```python
from build123d import *

# Parameters (mm, degrees)
SKETCH1_R           = 10
BOSS_EXTRUDE1_DEPTH = 10
SKETCH2_R           = 100
BOSS_EXTRUDE2_DEPTH = 10
SKETCH3_R           = 7.5
BOSS_EXTRUDE3_DEPTH = 10


with BuildPart() as part:
    # Sketch1 → Boss-Extrude1 (new body)
    with BuildSketch(Plane(origin=(0, 0, 0), x_dir=(1, 0, 0), z_dir=(0, 1, 0))):
        with BuildLine():
            ThreePointArc((48.173076923, 57.483516418), (-75, 0), (48.173076923, -57.483516418))
            ThreePointArc((48.173076923, -57.483516418), (30, 0), (48.173076923, 57.483516418))
        make_face()
        with Locations(Location((0, 0, 0), (0, 0, 270))):
            Circle(SKETCH1_R, mode=Mode.SUBTRACT)
    extrude(amount=BOSS_EXTRUDE1_DEPTH)

    # Sketch2 → Boss-Extrude2 (add)
    with BuildSketch(Plane.XZ):
        with Locations(Location((0, 0, 0), (0, 0, 270))):
            Circle(SKETCH2_R)
    extrude(amount=BOSS_EXTRUDE2_DEPTH)

    # Sketch3 → Boss-Extrude3 (add)
    with BuildSketch(Plane(origin=(0, 0, 0), x_dir=(1, 0, 0), z_dir=(0, 1, 0))):
        with Locations(Location((80, 0, 0), (0, 0, 90))):
            Circle(SKETCH3_R)
    extrude(amount=BOSS_EXTRUDE3_DEPTH)


solid = part.part
```
Verification items for the finished model (mm, model axes). A direction names the side the tool comes from. Round coordinates to 2 decimals unless told otherwise and drop trailing zeros. Order: outer loops, then holes, each group sorted by start corner. A loop starts at its lowest first (then second) coordinate and runs counter-clockwise, first axis right, second up. Notation, with made-up numbers: (39, 53.25) - (70, 53.25) arc R22 ccw to (70, 75.25) - close; hole circle Ø6 at (-34, 68.25). An arc over 180 degrees is marked (long way). Use CSV: the item, a comma, the result in double quotes. Start each with the question number.
1) Section check A-A, the plane y = 3.75. Record the cut outline in (x, z).
2) Mould release check, pull along Z, two halves, no side actions. Record for faces 3 (the flat face through (1, -10, 1)), 4 (the cylindrical face through (-74.962, 4.93, -2.381)), 5 (the cylindrical face through (30.004, 4.93, 0.857)): +Z half, -Z half, draft (parallel to the pull), parting line (faces both ways), or undercut.
3) Section check B-B, the plane x = 0. Record the cut outline in (y, z), plus the area to 3 significant figures.
4) Thickness scan on L1, parallel to X at y = 3.5, z = 0; L2, parallel to Y at x = 51, z = -18; L3, parallel to X at y = 6.25, z = 48. Record the ranges inside material, lowest first.
5) Go/stop test with flat-tipped pins: P1, Ø2, axis at y = -3.5, z = -48.5, coming from the +X side; P2, Ø5, axis at x = -52, y = -4.5, coming from the +Z side; P3, Ø6, axis at x = -6, y = 2, coming from the -Z side. Record where each tip stops, or that it passes through.
6) Access from +Z, -Z, +X, -X, +Y, -Y to the whole of each face (thin tool, end or side, straight path). Record for faces 1 (the flat face through (-14, 10, -1)), 2 (the cylindrical face through (86.654, 4.93, -3.461)).
7) Section check D-D, the plane x = 80. Record the cut outline in (y, z).
8) Section check C-C, the plane z = 34.5. Record the cut outline in (x, y).
Answers:
1,outline,"(48.17, -57.48) arc R100 cw to (48.17, 57.48) arc R75 ccw (long way) to start; circle Ø15 at (80, 0); hole circle Ø20 at (0, 0)"
2,face 3,"draft"
2,face 4,"parting line"
2,face 5,"undercut"
3,outline,"(-10, -100) - (0, -100) - (0, -75) - (10, -75) - (10, -10) - (0, -10) - (0, 10) - (10, 10) - (10, 75) - (0, 75) - (0, 100) - (-10, 100) - close"
3,area,"3,300 mm²"
4,L1,"x = -75 to -10, 10 to 30, 72.5 to 87.5"
4,L2,"y = -10 to 0"
4,L3,"x = -57.63 to 42.27"
5,P1,"stops at x = 88"
5,P2,"stops at z = 86.89"
5,P3,"stops at z = -99.93"
6,face 1,"+Z, -Z, +X, -X, +Y"
6,face 2,"+Y"
7,outline,"(-10, -60) - (0, -60) - (0, -7.5) - (10, -7.5) - (10, 7.5) - (0, 7.5) - (0, 60) - (-10, 60) - close"
8,outline,"(-93.86, -10) - (93.86, -10) - (93.86, 0) - (36.14, 0) - (36.14, 10) - (-66.59, 10) - (-66.59, 0) - (-93.86, 0) - close"
